The model under review builds one solid part; all positions refer to its coordinate system, in mm. A direction names the side the tool comes from. Give positions to 0.01 mm unless a question says otherwise; leave off trailing zeros. Loops run counter-clockwise (first coordinate to the right, second up) from the corner with the lowest first, then second, coordinate; pieces in that order, holes last. Notation, with made-up numbers: (26, -27.5) -> (79, -27.5) arc R38 ccw to (79, 11.5) -> close; hole circle Ø4 at (40, -32). An arc over 180 degrees is marked (long way). Write each question's results on one line, items separated by ' | '. Start each with the question number.
Q1. We need section D-D (y = -16). Write out the cut boundary in (x, z), plus the area to 3 significant figures.
Q2. Machinability: for faces 1 (the face through (17.8, -11.47, -8.81)), 2 (the face through (4.01, -18.06, -9.52)), 3 (the face through (-17.6, 11.8, -9.6)), which of the approach directions +Z, -Z, +X, -X, +Y, -Y give a long, thin tool a straight path to every point of the face, cutting with its end or side? Answer none if there is none.
Q3. We need section B-B (x = -6). Write out the cut boundary in (y, z).
Q4. Insertion check: pin 1 Ø7 at (x, y) = (-1, -21) entering from -Z; pin 2 Ø1 at (y, z) = (-37, -10) entering from -X; pin 3 Ø3 at (y, z) = (14.5, -9.5) entering from +X; pin 4 Ø5 at (x, y) = (19.49, -11.25) entering from -Z. Each pin has a flat end and moves straight along its axis. Give the tip position at first contact, or say it passes through.
Q5. We need section A-A (y = 0). Write out the cut boundary in (x, z), plus the area to 3 significant figures.
Q6. Wall thickness on L1, parallel to Y at x = -7, z = -8.7; L2, parallel to Y at x = 7.5, z = -10.95; L3, parallel to X at y = -11.25, z = -11.7: over which ranges is each line inside the solid? List them lowest first. Write a range as [from, to].
Q7. We need section C-C (x = 0). Give the number of separate pieces and of enclosed holes in the cut face, plus the area to 3 significant figures.
Q8. Mouldability with a two-part tool opening along X and no side actions: class faces 4 (the face through (-20.698, -34.829, -10.535)), 5 (the face through (13.887, -10.648, -12.014)), 6 (the face through (20.87, -34.03, -10.53)) as released by +X, released by -X, zero draft, split by the parting line, or undercut.
from build123d import *

# Parameters (mm, degrees)
SKETCH_2_R                   = 27.5
EXTRUDE_2_DEPTH              = 2
SKETCH_22_R                  = 10
CUT_EXTRUDE_1_DEPTH          = 2
FILLET_4_R                   = 0.2
SKETCH_54_R                  = 27.5
EXTRUDE_6_DEPTH              = 11
SKETCH_55_R                  = 18.5
CUT_EXTRUDE_2_DEPTH          = 8
HOLE_WIZARD_M4_1_D           = 4.5
HOLE_WIZARD_M4_1_CBORE_D     = 8
HOLE_WIZARD_M4_1_CBORE_DEPTH = 1
PATTERN_CIRCULAR_1_COUNT     = 3
SKETCH_59_R                  = 18.5
SKETCH_59_R_2                = 17.5
EXTRUDE_7_DEPTH              = 1
EXTRUDE_8_DEPTH              = 9
FILLET_6_R                   = 0.3
SKETCH_68_R                  = 9.5
CUT_EXTRUDE_7_DEPTH          = 7
SKETCH_69_R                  = 8.5
CUT_EXTRUDE_8_DEPTH          = 3
SKETCH_80_W                  = 72.028937147
SKETCH_80_H                  = 17.189961631
CUT_EXTRUDE_9_DEPTH          = 176.5
SKETCH_83_R                  = 18.5
SKETCH_83_R_2                = 17.5
EXTRUDE_9_DEPTH              = 2
PATTERN_CIRCULAR_2_COUNT     = 6


with BuildPart() as part:
    # 스케치2 → 보스-돌출2 (new body)
    with BuildSketch(Plane(origin=(0, 6, 0), x_dir=(1, 0, 0), z_dir=(0, 0, -1))):
        with Locations((0, 6)):
            Circle(SKETCH_2_R)
    extrude(amount=EXTRUDE_2_DEPTH)

    # 스케치22 → 컷-돌출1 (cut)
    with BuildSketch(Plane.XY):
        Circle(SKETCH_22_R)
    extrude(amount=-CUT_EXTRUDE_1_DEPTH, mode=Mode.SUBTRACT)

    # 필렛4
    fillet_4_edges = [part.edges().sort_by_distance(p)[0] for p in [
        (-10, 0, 0),
    ]]
    fillet(fillet_4_edges, radius=FILLET_4_R)

    # 스케치54 → 보스-돌출6 (add)
    with BuildSketch(Plane(origin=(0, 0, -2), x_dir=(-1, 0, 0), z_dir=(0, 0, -1))):
        Circle(SKETCH_54_R)
    extrude(amount=EXTRUDE_6_DEPTH)

    # 스케치55 → 컷-돌출2 (cut)
    with BuildSketch(Plane(origin=(0, 0, -13), x_dir=(-1, 0, 0), z_dir=(0, 0, -1))):
        Circle(SKETCH_55_R)
    extrude(amount=-CUT_EXTRUDE_2_DEPTH, mode=Mode.SUBTRACT)

    # M4 육각 소켓 머리 캡 나사용 카운터보어1 (through all)
    with Locations(Plane(origin=(0, 0, -5), x_dir=(-1, 0, 0), z_dir=(0, 0, -1))):
        with Locations((0, 6)):
            hole_wizard_m4_1 = CounterBoreHole(HOLE_WIZARD_M4_1_D / 2, HOLE_WIZARD_M4_1_CBORE_D / 2, HOLE_WIZARD_M4_1_CBORE_DEPTH)

    # 원형 패턴1: M4 육각 소켓 머리 캡 나사용 카운터보어1 ×3 about axis
    pattern_circular_1_axis = Axis((0, 0, 0), (0, 0, 1))
    for i in range(1, PATTERN_CIRCULAR_1_COUNT):
        add(hole_wizard_m4_1.rotate(pattern_circular_1_axis, i * 360 / PATTERN_CIRCULAR_1_COUNT), mode=Mode.SUBTRACT)

    # 스케치59 → 보스-돌출7 (add)
    with BuildSketch(Plane(origin=(0, 0, -5), x_dir=(-1, 0, 0), z_dir=(0, 0, -1))):
        Circle(SKETCH_59_R)
        Circle(SKETCH_59_R_2, mode=Mode.SUBTRACT)
    extrude(amount=EXTRUDE_7_DEPTH)

    # 스케치60 → 보스-돌출8 (add)
    with BuildSketch(Plane(origin=(0, 0, -13), x_dir=(-1, 0, 0), z_dir=(0, 0, -1))):
        with BuildLine():
            Line((-26.896591779, -5.729166667), (-14.670868243, -63.125))
            ThreePointArc((-14.670868243, -63.125), (0, -75), (14.670868243, -63.125))
            Line((14.670868243, -63.125), (26.896591779, -5.729166667))
            ThreePointArc((26.896591779, -5.729166667), (0, -27.5), (-26.896591779, -5.729166667))
        make_face()
    extrude(amount=-EXTRUDE_8_DEPTH)

    # 필렛6
    fillet_6_edges = [part.edges().sort_by_distance(p)[0] for p in [
        (18.5, 0, -6),
    ]]
    fillet(fillet_6_edges, radius=FILLET_6_R)

    # 스케치68 → 컷-돌출7 (cut)
    with BuildSketch(Plane.XY.offset(-4)):
        with Locations((0, -60)):
            Circle(SKETCH_68_R)
    extrude(amount=-CUT_EXTRUDE_7_DEPTH, mode=Mode.SUBTRACT)

    # 스케치69 → 컷-돌출8 (cut, through all)
    with BuildSketch(Plane.XY.offset(-11)):
        with Locations((0, -60)):
            Circle(SKETCH_69_R)
    extrude(amount=-CUT_EXTRUDE_8_DEPTH, mode=Mode.SUBTRACT)

    # 스케치80 → 컷-돌출9 (cut, symmetric)
    with BuildSketch(Plane(origin=(0, 0, 0), x_dir=(1, 0, 0), z_dir=(0, 1, 0))):
        with Locations((0.446829634, -0.594980816)):
            Rectangle(SKETCH_80_W, SKETCH_80_H)
    extrude(amount=CUT_EXTRUDE_9_DEPTH, both=True, mode=Mode.SUBTRACT)

    # 스케치83 → 보스-돌출9 (add)
    with BuildSketch(Plane(origin=(0, 0, -13), x_dir=(-1, 0, 0), z_dir=(0, 0, -1))):
        Circle(SKETCH_83_R)
        Circle(SKETCH_83_R_2, mode=Mode.SUBTRACT)
    extrude(amount=-EXTRUDE_9_DEPTH)

    # 스케치89 → M3 육각 소켓 머리 캡 나사용 카운터보어1 (revolve, cut)
    with BuildSketch(Plane(origin=(0, 22.5, -13), x_dir=(0, 1, 0), z_dir=(1, 0, 0))):
        Polygon((0, 0), (0, 223.021463052), (1.7, 222), (1.7, 3.4), (3.25, 3.4), (3.25, 0), align=None)
    hole_wizard_m3_1 = revolve(axis=Axis((0, 22.5, -19.35), (0, 0, 1)), mode=Mode.SUBTRACT)

    # 원형 패턴2: M3 육각 소켓 머리 캡 나사용 카운터보어1 ×6 about axis
    pattern_circular_2_axis = Axis((0, 0, 0), (0, 0, 1))
    for i in range(1, PATTERN_CIRCULAR_2_COUNT):
        add(hole_wizard_m3_1.rotate(pattern_circular_2_axis, i * 360 / PATTERN_CIRCULAR_2_COUNT), mode=Mode.SUBTRACT)


solid = part.part
Output:
1) outline: (-24.71, -13) -> (-7.09, -13) -> (-7.09, -11) -> (-9.29, -11) -> (-9.29, -8) -> (-24.71, -8) -> close; (7.09, -13) -> (24.71, -13) -> (24.71, -8) -> (9.29, -8) -> (9.29, -11) -> (7.09, -11) -> close | area: 163 mm2
2) face 1: +Z, -Z | face 2: +Z | face 3: -Z
3) outline: (-73.75, -13) -> (-66.02, -13) -> (-66.02, -11) -> (-67.37, -11) -> (-67.37, -8) -> (-73.75, -8) -> close; (-53.98, -13) -> (-16.44, -13) -> (-16.44, -11) -> (-17.5, -11) -> (-17.5, -8) -> (-52.63, -8) -> (-52.63, -11) -> (-53.98, -11) -> close; (16.44, -13) -> (26.84, -13) -> (26.84, -8) -> (17.5, -8) -> (17.5, -11) -> (16.44, -11) -> close
4) pin 1: z = -13 | pin 2: x = -20.34 | pin 3: x = 24.23 | pin 4: z = -9.6
5) outline: (-27.5, -13) -> (-17.5, -13) -> (-17.5, -11) -> (-18.5, -11) -> (-18.5, -8) -> (-27.5, -8) -> close; (17.5, -13) -> (27.5, -13) -> (27.5, -8) -> (18.5, -8) -> (18.5, -11) -> (17.5, -11) -> close | area: 94.0 mm2
6) L1: [-73.27, -66.42], [-53.58, -17.12], [17.12, 26.59] | L2: [-72.99, -65.83], [-54.17, -16.91], [16.91, 26.46] | L3: [-25.72, -22.74], [-16.24, -13.4], [13.4, 16.24], [22.74, 25.72]
7) separate pieces: 5 | enclosed holes: 0 | area: 185 mm2
8) face 4: released by -X | face 5: undercut | face 6: released by +X
